Can you work these out from the model? Positions are in its coordinate system, mm. A direction names the side the tool comes from. Coordinates: 2 decimals unless noted, no trailing zeros. Order: outer loops, then holes, each group sorted by start corner. A loop starts at its lowest first (then second) coordinate and runs counter-clockwise, first axis right, second up. Notation, with made-up numbers: (21.25, 71.5) -> (63.25, 71.5) arc R9 ccw to (63.25, 88.5) -> close; hole circle Ø4 at (-8.5, 68.25). An arc over 180 degrees is marked (long way). Write item = value, one per line.
```python
from build123d import *

# Parameters (mm, degrees)
F0_W      = 107.95
F0_H      = 63.5
F1_DEPTH  = 57.15
F2_W      = 6.35
F2_H      = 6.35
F3_DEPTH  = 57.151
F4_W      = 12.7
F4_H      = 63.5
F5_DEPTH  = 57.151
F7_DEPTH  = 63.501
F9_DEPTH  = 38.1
F11_DEPTH = 25.4
F12_R     = 6.35
F13_DEPTH = 25.4


with BuildPart() as f1:
    # F0 (on Front) → F1 (new body)
    with BuildSketch(Plane.XZ):
        with Locations((53.975, 31.75)):
            Rectangle(F0_W, F0_H)
    extrude(amount=F1_DEPTH)

    # F2 (on face) → F3 (cut, through all)
    with BuildSketch(Plane.XZ.offset(57.15)):
        with Locations((3.175, 3.175)):
            Rectangle(F2_W, F2_H)
    extrude(amount=-F3_DEPTH, mode=Mode.SUBTRACT)

    # F4 (on face) → F5 (cut, through all)
    with BuildSketch(Plane.XZ.offset(57.15)):
        with Locations((101.6, 31.75)):
            Rectangle(F4_W, F4_H)
    extrude(amount=-F5_DEPTH, mode=Mode.SUBTRACT)

    # F6 (on face) → F7 (cut, through all)
    with BuildSketch(Plane.XY.offset(63.5)):
        Polygon((95.25, -15.875), (95.25, 0), (79.375, 0), align=None)
    extrude(amount=-F7_DEPTH, mode=Mode.SUBTRACT)

    # F8 (on face) → F9 (cut)
    with BuildSketch(Plane.XZ.offset(57.15)):
        Polygon((95.25, 63.5), (0, 63.5), (0, 31.75), (44.45, 31.75), (44.45, 19.05), (57.15, 19.05), (57.15, 12.7), (44.45, 12.7), (44.45, 0), (95.25, 0), align=None)
    extrude(amount=-F9_DEPTH, mode=Mode.SUBTRACT)

    # F10 (on face) → F11 (cut)
    with BuildSketch(Plane.XZ.offset(19.05)):
        Polygon((95.25, 19.05), (95.25, 63.5), (50.8, 63.5), align=None)
    extrude(amount=-F11_DEPTH, mode=Mode.SUBTRACT)

    # F12 (on face) → F13 (cut)
    with BuildSketch(Plane.XZ.offset(19.05)):
        with Locations((19.05, 50.8)):
            Circle(F12_R)
    extrude(amount=-F13_DEPTH, mode=Mode.SUBTRACT)


solid = f1.part
```
Item 1: I want a section at D-D, the plane y = -13.5. Please give me the cut outline in (x, z) (3 decimals).
A:
outline = (0, 6.35) -> (6.35, 6.35) -> (6.35, 0) -> (92.875, 0) -> (92.875, 21.425) -> (50.8, 63.5) -> (0, 63.5) -> close; hole circle Ø12.7 at (19.05, 50.8)
Item 2: For faces 1 (the flat face through (40, -22, 0)), 2 (the flat face through (51, -38, 12.7)), 3 (the flat face through (6.35, -29, 3)), 4 (the flat face through (51, -38, 19.05)), 5 (the flat face through (22, -38, 31.75)), which set-ups out of +Z, -Z, +X, -X, +Y, -Y let a thin tool reach every point of the face, with its end or its side?
A:
face_1 = -Z, +X, -X, +Y, -Y
face_2 = -Z, +X, -Y
face_3 = -Z, -X, +Y, -Y
face_4 = +Z, +X, -Y
face_5 = +Z, +X, -X, -Y
Item 3: If we mould it in two halves opening along Z, with no side actions, what happens to faces 6 (the cylindrical face through (22.464, -9.658, 56.154)), 7 (the flat face through (57.15, -38, 16)), 8 (the flat face through (25, -9, 63.5))? For each: pulls with the +Z half, pulls with the -Z half, needs draft (parallel to the pull), parting line crosses it, or undercut.
A:
face_6 = undercut
face_7 = needs draft
face_8 = pulls with the +Z half
Item 4: I'm going to push flat-ended pins straight in: P1, Ø10, axis at x = 50, y = -39, coming from the +Z side; P2, Ø4, axis at x = 51, y = -37.5, coming from the -Z side; P3, Ø14.5, axis at x = 19.05, z = 50.8, coming from the -Y side. Where does each tip first touch, or does it pass through?
A:
P1 = 19.05
P2 = 12.7
P3 = -19.05
Item 5: I want a section at A-A, the plane z = 50.8. Please give me the cut outline in (x, y), plus the area to 3 significant figures.
A:
outline = (0, -19.05) -> (12.7, -19.05) -> (12.7, 0) -> (0, 0) -> close; (25.4, -19.05) -> (63.5, -19.05) -> (63.5, 0) -> (25.4, 0) -> close
area = 968 mm2
Item 6: I want a section at B-B, the plane x = 19.05. Please give me the cut outline in (y, z).
A:
outline = (-57.15, 0) -> (0, 0) -> (0, 44.45) -> (-19.05, 44.45) -> (-19.05, 31.75) -> (-57.15, 31.75) -> close; (-19.05, 57.15) -> (0, 57.15) -> (0, 63.5) -> (-19.05, 63.5) -> close
Item 7: I want a section at C-C, the plane y = -36.5. Please give me the cut outline in (x, z).
A:
outline = (0, 6.35) -> (6.35, 6.35) -> (6.35, 0) -> (44.45, 0) -> (44.45, 12.7) -> (57.15, 12.7) -> (57.15, 19.05) -> (44.45, 19.05) -> (44.45, 31.75) -> (0, 31.75) -> close
Item 8: If I drill on probe 1 along Y at (x, z) = (55, 12); probe 2 along Z at (x, y) = (19.05, -14); probe 3 along Z at (x, y) = (50.5, -43.5), over which ranges is the centre line in solid material (lowest first)?
A:
probe_1 = -19.05 to 0
probe_2 = 0 to 44.45, 57.15 to 63.5
probe_3 = 12.7 to 19.05
